```python
from build123d import *

# Parameters (mm, degrees)
SKETCH1_W           = 38
SKETCH1_H           = 20
BOSS_EXTRUDE1_DEPTH = 1.6
SKETCH2_R           = 1.125
CUT_EXTRUDE1_DEPTH  = 2.6
SKETCH3_R           = 0.5
CUT_EXTRUDE2_DEPTH  = 2.6


with BuildPart() as part:
    # Sketch1 → Boss-Extrude1 (new body)
    with BuildSketch(Plane(origin=(0, 0, 0), x_dir=(1, 0, 0), z_dir=(0, 1, 0))):
        with Locations((19, 10)):
            Rectangle(SKETCH1_W, SKETCH1_H)
    extrude(amount=BOSS_EXTRUDE1_DEPTH)

    # Sketch2 → Cut-Extrude1 (cut, through all)
    with BuildSketch(Plane(origin=(0, 1.6, 0), x_dir=(1, 0, 0), z_dir=(0, 1, 0))):
        with Locations((2.1, 18)):
            Circle(SKETCH2_R)
        with Locations((2.1, 2)):
            Circle(SKETCH2_R)
    extrude(amount=-CUT_EXTRUDE1_DEPTH, mode=Mode.SUBTRACT)

    # Sketch3 → Cut-Extrude2 (cut, through all)
    with BuildSketch(Plane(origin=(0, 1.6, 0), x_dir=(1, 0, 0), z_dir=(0, 1, 0))):
        with Locations((5.6, 16.35)):
            Circle(SKETCH3_R)
        with Locations((8.14, 16.35)):
            Circle(SKETCH3_R)
        with Locations((10.68, 16.35)):
            Circle(SKETCH3_R)
        with Locations((13.22, 16.35)):
            Circle(SKETCH3_R)
        with Locations((15.76, 16.35)):
            Circle(SKETCH3_R)
        with Locations((18.3, 16.35)):
            Circle(SKETCH3_R)
        with Locations((20.84, 16.35)):
            Circle(SKETCH3_R)
        with Locations((23.38, 16.35)):
            Circle(SKETCH3_R)
        with Locations((25.92, 16.35)):
            Circle(SKETCH3_R)
        with Locations((28.46, 16.35)):
            Circle(SKETCH3_R)
        with Locations((31, 16.35)):
            Circle(SKETCH3_R)
        with Locations((33.54, 16.35)):
            Circle(SKETCH3_R)
        with Locations((36.08, 16.35)):
            Circle(SKETCH3_R)
        with Locations((8.14, 13.81)):
            Circle(SKETCH3_R)
        with Locations((10.68, 13.81)):
            Circle(SKETCH3_R)
        with Locations((13.22, 13.81)):
            Circle(SKETCH3_R)
        with Locations((15.76, 13.81)):
            Circle(SKETCH3_R)
        with Locations((18.3, 13.81)):
            Circle(SKETCH3_R)
        with Locations((20.84, 13.81)):
            Circle(SKETCH3_R)
        with Locations((23.38, 13.81)):
            Circle(SKETCH3_R)
        with Locations((25.92, 13.81)):
            Circle(SKETCH3_R)
        with Locations((28.46, 13.81)):
            Circle(SKETCH3_R)
        with Locations((31, 13.81)):
            Circle(SKETCH3_R)
        with Locations((33.54, 13.81)):
            Circle(SKETCH3_R)
        with Locations((36.08, 13.81)):
            Circle(SKETCH3_R)
        with Locations((8.14, 11.27)):
            Circle(SKETCH3_R)
        with Locations((10.68, 11.27)):
            Circle(SKETCH3_R)
        with Locations((13.22, 11.27)):
            Circle(SKETCH3_R)
        with Locations((15.76, 11.27)):
            Circle(SKETCH3_R)
        with Locations((18.3, 11.27)):
            Circle(SKETCH3_R)
        with Locations((20.84, 11.27)):
            Circle(SKETCH3_R)
        with Locations((23.38, 11.27)):
            Circle(SKETCH3_R)
        with Locations((25.92, 11.27)):
            Circle(SKETCH3_R)
        with Locations((28.46, 11.27)):
            Circle(SKETCH3_R)
        with Locations((31, 11.27)):
            Circle(SKETCH3_R)
        with Locations((33.54, 11.27)):
            Circle(SKETCH3_R)
        with Locations((36.08, 11.27)):
            Circle(SKETCH3_R)
        with Locations((8.14, 8.73)):
            Circle(SKETCH3_R)
        with Locations((10.68, 8.73)):
            Circle(SKETCH3_R)
        with Locations((13.22, 8.73)):
            Circle(SKETCH3_R)
        with Locations((15.76, 8.73)):
            Circle(SKETCH3_R)
        with Locations((18.3, 8.73)):
            Circle(SKETCH3_R)
        with Locations((20.84, 8.73)):
            Circle(SKETCH3_R)
        with Locations((23.38, 8.73)):
            Circle(SKETCH3_R)
        with Locations((25.92, 8.73)):
            Circle(SKETCH3_R)
        with Locations((28.46, 8.73)):
            Circle(SKETCH3_R)
        with Locations((31, 8.73)):
            Circle(SKETCH3_R)
        with Locations((33.54, 8.73)):
            Circle(SKETCH3_R)
        with Locations((36.08, 8.73)):
            Circle(SKETCH3_R)
        with Locations((8.14, 6.19)):
            Circle(SKETCH3_R)
        with Locations((10.68, 6.19)):
            Circle(SKETCH3_R)
        with Locations((13.22, 6.19)):
            Circle(SKETCH3_R)
        with Locations((15.76, 6.19)):
            Circle(SKETCH3_R)
        with Locations((18.3, 6.19)):
            Circle(SKETCH3_R)
        with Locations((20.84, 6.19)):
            Circle(SKETCH3_R)
        with Locations((23.38, 6.19)):
            Circle(SKETCH3_R)
        with Locations((25.92, 6.19)):
            Circle(SKETCH3_R)
        with Locations((28.46, 6.19)):
            Circle(SKETCH3_R)
        with Locations((31, 6.19)):
            Circle(SKETCH3_R)
        with Locations((33.54, 6.19)):
            Circle(SKETCH3_R)
        with Locations((36.08, 6.19)):
            Circle(SKETCH3_R)
        with Locations((8.14, 3.65)):
            Circle(SKETCH3_R)
        with Locations((10.68, 3.65)):
            Circle(SKETCH3_R)
        with Locations((13.22, 3.65)):
            Circle(SKETCH3_R)
        with Locations((15.76, 3.65)):
            Circle(SKETCH3_R)
        with Locations((18.3, 3.65)):
            Circle(SKETCH3_R)
        with Locations((20.84, 3.65)):
            Circle(SKETCH3_R)
        with Locations((23.38, 3.65)):
            Circle(SKETCH3_R)
        with Locations((25.92, 3.65)):
            Circle(SKETCH3_R)
        with Locations((28.46, 3.65)):
            Circle(SKETCH3_R)
        with Locations((31, 3.65)):
            Circle(SKETCH3_R)
        with Locations((33.54, 3.65)):
            Circle(SKETCH3_R)
        with Locations((36.08, 3.65)):
            Circle(SKETCH3_R)
        with Locations((5.6, 13.81)):
            Circle(SKETCH3_R)
        with Locations((5.6, 11.27)):
            Circle(SKETCH3_R)
        with Locations((5.6, 8.73)):
            Circle(SKETCH3_R)
        with Locations((5.6, 6.19)):
            Circle(SKETCH3_R)
        with Locations((5.6, 3.65)):
            Circle(SKETCH3_R)
    extrude(amount=-CUT_EXTRUDE2_DEPTH, mode=Mode.SUBTRACT)


solid = part.part
```
Geometry check sheet. Reference: the model listing, model coordinates, mm. Give positions to 0.01 mm unless a question says otherwise; leave off trailing zeros. Loops run counter-clockwise (first coordinate to the right, second up) from the corner with the lowest first, then second, coordinate; pieces in that order, holes last. Notation, with made-up numbers: M 12.25,6.25 L 17.25,6.25 A22 cw 17.25,39.25 Z; hole C 15.5,40.5 d3. An arc over 180 degrees is marked long. Write item = value, one per line. Start each with the question number.
1. Section check B-B, the plane z = -18. Enter the section's corners in (x, y) (3 decimals), plus the area to 3 significant figures.
2. Go/stop test with a flat-tipped pin: P1, Ø1.8, axis at x = 2.1, z = -2, coming from the +Y side. Record where the tip stops, or that it passes through.
3. Draft check along X on faces 1 (the face through (33.432, 0.811, -15.862)), 2 (the face through (19, 1.6, -10)). Enter one of: +X half, -X half, draft (parallel to the pull), parting line (faces both ways), or undercut.
4. Section check C-C, the plane y = 0.4. Give the number of separate pieces and of enclosed holes in the cut face, plus the area to 3 significant figures.
5. Thickness scan on probe 1 along X at (y, z) = (1.05, -2) (3 decimals); probe 2 along X at (y, z) = (0.65, -3). Record the ranges inside material, lowest first.
6. Section check A-A, the plane x = 20.84. Enter the section's corners in (y, z), plus the area to 3 significant figures.
Values follow:
q1.outline = M 0,0 L 0.975,0 L 0.975,1.6 L 0,1.6 Z; M 3.225,0 L 38,0 L 38,1.6 L 3.225,1.6 Z
q1.area = 57.2 mm^2
q2.P1 = through
q3.face_1 = undercut
q3.face_2 = draft
q4.separate_pieces = 1
q4.enclosed_holes = 80
q4.area = 691 mm^2
q5.probe_1 = 0 to 0.975, 3.225 to 38
q5.probe_2 = 0 to 1.58, 2.62 to 38
q6.outline = M 0,-20 L 1.6,-20 L 1.6,-16.85 L 0,-16.85 Z; M 0,-15.85 L 1.6,-15.85 L 1.6,-14.31 L 0,-14.31 Z; M 0,-13.31 L 1.6,-13.31 L 1.6,-11.77 L 0,-11.77 Z; M 0,-10.77 L 1.6,-10.77 L 1.6,-9.23 L 0,-9.23 Z; M 0,-8.23 L 1.6,-8.23 L 1.6,-6.69 L 0,-6.69 Z; M 0,-5.69 L 1.6,-5.69 L 1.6,-4.15 L 0,-4.15 Z; M 0,-3.15 L 1.6,-3.15 L 1.6,0 L 0,0 Z
q6.area = 22.4 mm^2
